from build123d import *

# Parameters (mm, degrees)
BOSS_EXTRUDE1_DEPTH      = 10
BOSS_EXTRUDE2_DEPTH      = 30
BOSS_EXTRUDE2_DEPTH_BACK = 20
SKETCH3_W                = 20
SKETCH3_H                = 25
BOSS_EXTRUDE3_DEPTH      = 3
SKETCH4_W                = 20
SKETCH4_H                = 3
BOSS_EXTRUDE4_DEPTH      = 8
SKETCH5_R                = 1.5
CUT_EXTRUDE1_DEPTH       = 49.09105946
SKETCH5_3_R              = 2.5
SKETCH5_3_R_2            = 1.5
CUT_EXTRUDE2_DEPTH       = 2
SKETCH6_R                = 1.5
CUT_EXTRUDE3_DEPTH       = 6.5
SKETCH6_3_R              = 2.5
SKETCH6_3_R_2            = 1.5
CUT_EXTRUDE4_DEPTH       = 3
MOVE_FACE1_BY            = 0.2
MOVE_FACE1_2_BY          = 0.2
MOVE_FACE1_3_BY          = 0.2
MOVE_FACE1_4_BY          = 0.2
MOVE_FACE1_5_BY          = 0.2
MOVE_FACE1_6_BY          = 0.2
MOVE_FACE1_7_BY          = 0.2
MOVE_FACE1_8_BY          = 0.2
MOVE_FACE1_9_BY          = 0.2
MOVE_FACE1_10_BY         = 0.2
MOVE_FACE1_11_BY         = 0.2
MOVE_FACE1_12_BY         = 0.2
MOVE_FACE1_13_BY         = 0.2
MOVE_FACE1_14_BY         = 0.2


with BuildPart() as part:
    # Sketch1 → Boss-Extrude1 (new, symmetric)
    with BuildSketch(Plane.XY):
        Polygon((0, -7.5), (-32, -7.5), (-32, 7.5), (-12, 7.5), (-12, 12.5), (0, 12.5), align=None)
    extrude(amount=BOSS_EXTRUDE1_DEPTH, both=True)

    # Sketch2 → Boss-Extrude2 (add, two sides)
    with BuildSketch(Plane(origin=(0, 0, 0), x_dir=(1, 0, 0), z_dir=(0, 1, 0))) as boss_extrude2_sk:
        Polygon((-32, 13.5), (-35.5, 13.5), (-35.5, -13.5), (-32, -13.5), (-32, -10), (-29, -10), (-29, 10), (-32, 10), align=None)
    extrude(amount=BOSS_EXTRUDE2_DEPTH)
    extrude(boss_extrude2_sk.sketch, amount=-BOSS_EXTRUDE2_DEPTH_BACK)

    # Sketch3 → Boss-Extrude3 (add)
    with BuildSketch(Plane(origin=(0, 12.5, 0), x_dir=(1, 0, 0), z_dir=(0, 1, 0))):
        with Locations((-2, 0)):
            Rectangle(SKETCH3_W, SKETCH3_H)
    extrude(amount=BOSS_EXTRUDE3_DEPTH)

    # Sketch4 → Boss-Extrude4 (add)
    with BuildSketch(Plane(origin=(0, 0, 0), x_dir=(0, 0, -1), z_dir=(1, 0, 0))):
        with Locations((0, 11)):
            Rectangle(SKETCH4_W, SKETCH4_H)
    extrude(amount=BOSS_EXTRUDE4_DEPTH)

    # Sketch5 → Cut-Extrude1 (cut, through all)
    with BuildSketch(Plane.XZ.offset(-9.5)):
        with Locations((4, 0)):
            Circle(SKETCH5_R)
    extrude(amount=-CUT_EXTRUDE1_DEPTH, mode=Mode.SUBTRACT)

    # Sketch5<3> → Cut-Extrude2 (cut)
    with BuildSketch(Plane.XZ.offset(-9.5)):
        with Locations((4, 0)):
            Circle(SKETCH5_3_R)
        with Locations((4, 0)):
            Circle(SKETCH5_3_R_2, mode=Mode.SUBTRACT)
    extrude(amount=-CUT_EXTRUDE2_DEPTH, mode=Mode.SUBTRACT)

    # Sketch6 → Cut-Extrude3 (cut)
    with BuildSketch(Plane(origin=(-29, 0, 0), x_dir=(0, 0, -1), z_dir=(1, 0, 0))):
        with Locations((0, 18.75)):
            Circle(SKETCH6_R)
    extrude(amount=-CUT_EXTRUDE3_DEPTH, mode=Mode.SUBTRACT)

    # Sketch6<3> → Cut-Extrude4 (cut)
    with BuildSketch(Plane(origin=(-29, 0, 0), x_dir=(0, 0, -1), z_dir=(1, 0, 0))):
        with Locations((0, 18.75)):
            Circle(SKETCH6_3_R)
        with Locations((0, 18.75)):
            Circle(SKETCH6_3_R_2, mode=Mode.SUBTRACT)
    extrude(amount=-CUT_EXTRUDE4_DEPTH, mode=Mode.SUBTRACT)

    # Move Face1: a face moved inward by 0.2
    extrude(part.faces().sort_by_distance((7.2, 9.5, 0))[0], amount=MOVE_FACE1_BY, dir=(0, 1, 0), mode=Mode.SUBTRACT)

    # Move Face1 2: a face moved inward by 0.2
    extrude(part.faces().sort_by_distance((-29, 24.375, 0))[0], amount=MOVE_FACE1_2_BY, dir=(-1, 0, 0), mode=Mode.SUBTRACT)

    # Move Face1 3: a face moved inward by 0.2
    extrude(part.faces().sort_by_distance((-2, 12.5, -11.25))[0], amount=MOVE_FACE1_3_BY, dir=(0, 1, 0), mode=Mode.SUBTRACT)

    # Move Face1 4: a face moved inward by 0.2
    extrude(part.faces().sort_by_distance((-2, 14, -12.5))[0], amount=MOVE_FACE1_4_BY, dir=(0, 0, 1), mode=Mode.SUBTRACT)

    # Move Face1 5: a face moved inward by 0.2
    extrude(part.faces().sort_by_distance((-2.086039354, 15.5, 0))[0], amount=MOVE_FACE1_5_BY, dir=(0, -1, 0), mode=Mode.SUBTRACT)

    # Move Face1 6: a face moved inward by 0.2
    extrude(part.faces().sort_by_distance((-2, 14, 12.5))[0], amount=MOVE_FACE1_6_BY, dir=(0, 0, -1), mode=Mode.SUBTRACT)

    # Move Face1 7: a face moved inward by 0.2
    extrude(part.faces().sort_by_distance((-2, 12.5, 11.25))[0], amount=MOVE_FACE1_7_BY, dir=(0, 1, 0), mode=Mode.SUBTRACT)

    # Move Face1 8: a face moved inward by 0.2
    extrude(part.faces().sort_by_distance((-33.75, 5, -13.5))[0], amount=MOVE_FACE1_8_BY, dir=(0, 0, 1), mode=Mode.SUBTRACT)

    # Move Face1 9: a face moved inward by 0.2
    extrude(part.faces().sort_by_distance((-32, 5, -11.75))[0], amount=MOVE_FACE1_9_BY, dir=(-1, 0, 0), mode=Mode.SUBTRACT)

    # Move Face1 10: a face moved inward by 0.2
    extrude(part.faces().sort_by_distance((-16.661434978, 2.412556054, -10))[0], amount=MOVE_FACE1_10_BY, dir=(0, 0, 1), mode=Mode.SUBTRACT)

    # Move Face1 11: a face moved inward by 0.2
    extrude(part.faces().sort_by_distance((-35.5, 4.92762622, 0))[0], amount=MOVE_FACE1_11_BY, dir=(1, 0, 0), mode=Mode.SUBTRACT)

    # Move Face1 12: a face moved inward by 0.2
    extrude(part.faces().sort_by_distance((-16.661434978, 2.412556054, 10))[0], amount=MOVE_FACE1_12_BY, dir=(0, 0, -1), mode=Mode.SUBTRACT)

    # Move Face1 13: a face moved inward by 0.2
    extrude(part.faces().sort_by_distance((-32, 5, 11.75))[0], amount=MOVE_FACE1_13_BY, dir=(-1, 0, 0), mode=Mode.SUBTRACT)

    # Move Face1 14: a face moved inward by 0.2
    extrude(part.faces().sort_by_distance((-33.75, 5, 13.5))[0], amount=MOVE_FACE1_14_BY, dir=(0, 0, -1), mode=Mode.SUBTRACT)


solid = part.part
Read the model definition and answer for the solid it produces. Units are mm, in the model's axes. A direction names the side the tool comes from. Give positions to 0.01 mm unless a question says otherwise; leave off trailing zeros. Write each loop counter-clockwise with the first axis right and the second up, starting at its lowest first coordinate (ties: lowest second). Pieces come first, ordered by that corner, then holes. Notation, with made-up numbers: (22, 25.25) - (56, 25.25) arc R14 cw to (56, 40.25) - close; hole circle Ø6 at (27.5, -19.5). An arc over 180 degrees is marked (long way). Use CSV: the item, a comma, the result in double quotes. Start each with the question number.
Item 1: For faces 1 (the flat face through (-29.2, 16, 0)), 2 (the flat face through (-2, 12.7, -11)), 3 (the flat face through (-29, -14, 0)), determine the directions among +Z, -Z, +X, -X, +Y, -Y from which every point of the face is accessible in a straight line to the end or side of a thin tool.
Item 2: The part is cut by section B-B, the plane z = -4.75. Give the vertices of the cut face in (x, y).
Item 3: The part is cut by section C-C, the plane x = 4. Give the vertices of the cut face in (y, z).
Item 4: Consider line 1 (Z direction, x = 4, y = 10.95); line 2 (Z direction, x = 4, y = 13.35); line 3 (Y direction, x = -33.55, z = 0). Determine where each line is inside the solid, lowest interval first.
Item 5: The mould has two halves that part along Z. Classify faces 4 (the flat face through (-34, 5, 13.3)), 5 (the flat face through (-32, 17, 0)), 6 (the cylindrical face through (-33.627, 20.237, 0.195)), 7 (the flat face through (-32, 30, 0)): pulls with the +Z half, pulls with the -Z half, needs draft (parallel to the pull), parting line crosses it, or undercut.
Item 6: The part is cut by section A-A, the plane y = 18.75. Give the vertices of the cut face in (x, z).
Item 7: Flat-ended cylindrical pins translate along their axes: P1, Ø3, axis at x = 2, y = 13.5, coming from the +Z side; P2, Ø6, axis at y = 18.75, z = 0, coming from the +X side; P3, Ø1.8, axis at y = 3, z = 11.5, coming from the +X side. Find the tip coordinate at first contact, or state that the pin passes through.
Item 8: The part is cut by section D-D, the plane y = 24. Give the vertices of the cut face in (x, z).
Taken from the geometry:
1,face 1,"+Z, -Z, +Y"
1,face 2,"-Z, +X, -Y"
1,face 3,"+Z, -Z, +X, -Y"
2,outline,"(-35.3, -20) - (-29, -20) - (-29, -7.5) - (0, -7.5) - (0, 9.7) - (8, 9.7) - (8, 15.3) - (-12, 15.3) - (-12, 7.5) - (-29.2, 7.5) - (-29.2, 30) - (-35.3, 30) - close"
3,outline,"(9.7, -9.8) - (12.7, -9.8) - (12.7, -12.3) - (15.3, -12.3) - (15.3, -1.5) - (11.5, -1.5) - (11.5, -2.5) - (9.7, -2.5) - close; (9.7, 2.5) - (11.5, 2.5) - (11.5, 1.5) - (15.3, 1.5) - (15.3, 12.3) - (12.7, 12.3) - (12.7, 9.8) - (9.7, 9.8) - close"
4,line 1,"-9.8 to -2.5, 2.5 to 9.8"
4,line 2,"-12.3 to -1.5, 1.5 to 12.3"
4,line 3,"-20 to 17.25, 20.25 to 30"
5,face 4,"pulls with the +Z half"
5,face 5,"undercut"
5,face 6,"undercut"
5,face 7,"needs draft"
6,outline,"(-35.3, -13.3) - (-32.2, -13.3) - (-32.2, -9.8) - (-29.2, -9.8) - (-29.2, -2.5) - (-32, -2.5) - (-32, -1.5) - (-35.3, -1.5) - close; (-35.3, 1.5) - (-32, 1.5) - (-32, 2.5) - (-29.2, 2.5) - (-29.2, 9.8) - (-32.2, 9.8) - (-32.2, 13.3) - (-35.3, 13.3) - close"
7,P1,"z = 12.3"
7,P2,"x = -29.2"
7,P3,"x = -32.2"
8,outline,"(-35.3, -13.3) - (-32.2, -13.3) - (-32.2, -9.8) - (-29.2, -9.8) - (-29.2, 9.8) - (-32.2, 9.8) - (-32.2, 13.3) - (-35.3, 13.3) - close"
